Verification items for the finished model (mm, model axes). Face numbers are marked on the shaded views. A direction names the side the tool comes from. Round coordinates to 2 decimals unless told otherwise and drop trailing zeros. Write each loop counter-clockwise with the first axis right and the second up, starting at its lowest first coordinate (ties: lowest second). Pieces come first, ordered by that corner, then holes. Notation, with made-up numbers: (50, 38.5) - (83, 38.5) arc R13 ccw to (83, 51.5) - close; hole circle Ø1 at (74.5, -20). An arc over 180 degrees is marked (long way). Write each question's results on one line, items separated by ' | '.
```python
from build123d import *

# Parameters (mm, degrees)
SKETCH1_W           = 31
SKETCH1_H           = 26
BOSS_EXTRUDE1_DEPTH = 16.5
CUT_EXTRUDE1_START  = -6.5
SKETCH3_R           = 1.715784354
CUT_EXTRUDE1_DEPTH  = 8
SKETCH4_W           = 7.501797644
SKETCH4_H           = 16.91664374
CUT_EXTRUDE2_DEPTH  = 14.5


with BuildPart() as part:
    # Sketch1 → Boss-Extrude1 (new body)
    with BuildSketch(Plane.XY):
        with Locations((15.5, 13)):
            Rectangle(SKETCH1_W, SKETCH1_H)
    extrude(amount=BOSS_EXTRUDE1_DEPTH)

    # Sketch3 → Cut-Extrude1 (cut)
    with BuildSketch(Plane.XY.offset(16.5).offset(CUT_EXTRUDE1_START)):
        Polygon((0, 0), (0, 4.632335589), (6.323496347, 4.632335589), (6.323496347, 21.367664411), (0, 21.367664411), (0, 26), (31, 26), (31, 0), align=None)
        with Locations((3.010252107, 2.158101323)):
            Circle(SKETCH3_R, mode=Mode.SUBTRACT)
        with Locations((19.83045716, 2.158101323)):
            Circle(SKETCH3_R, mode=Mode.SUBTRACT)
        with Locations(Location((3.010252107, 23.841898677, 0), (0, 0, 180))):
            Circle(SKETCH3_R, mode=Mode.SUBTRACT)
        with Locations(Location((19.83045716, 23.841898677, 0), (0, 0, 180))):
            Circle(SKETCH3_R, mode=Mode.SUBTRACT)
    extrude(amount=-CUT_EXTRUDE1_DEPTH, mode=Mode.SUBTRACT)

    # Sketch4 → Cut-Extrude2 (cut)
    with BuildSketch(Plane.XY.offset(16.5)):
        with Locations((3.750898822, 13)):
            Rectangle(SKETCH4_W, SKETCH4_H)
    extrude(amount=-CUT_EXTRUDE2_DEPTH, mode=Mode.SUBTRACT)


solid = part.part
```
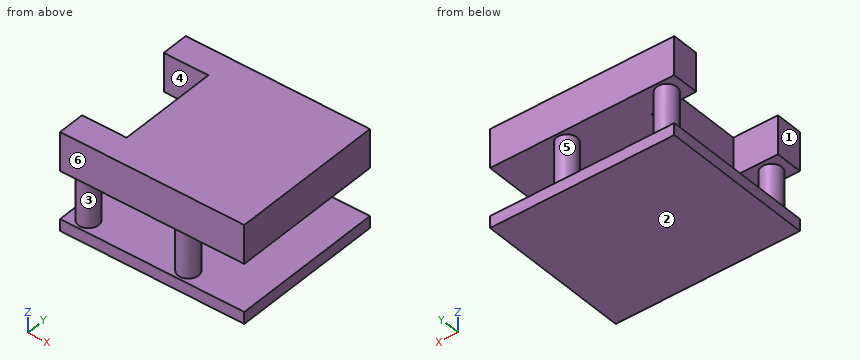
(1) Mould release check, pull along Z, two halves, no side actions. Record for the marked faces 1, 2 and 3: released by +Z, released by -Z, zero draft, split by the parting line, or undercut.
Answer:
face 1: zero draft | face 2: released by -Z | face 3: undercut
(2) Section check D-D (z = 12.25). Record the cut outline in (x, y).
Answer:
outline: (0, 0) - (31, 0) - (31, 26) - (0, 26) - (0, 21.46) - (7.5, 21.46) - (7.5, 4.54) - (0, 4.54) - close
(3) Section check C-C (x = 28). Record the cut outline in (y, z).
Answer:
outline: (0, 0) - (26, 0) - (26, 2) - (0, 2) - close; (0, 10) - (26, 10) - (26, 16.5) - (0, 16.5) - close
(4) Go/stop test with flat-tipped pins: pin 1 Ø1.5 at (x, z) = (25, 3.5) entering from +Y; pin 2 Ø2 at (y, z) = (10.5, 11.5) entering from -X. Record where each tip stops, or that it passes through.
Answer:
pin 1: through | pin 2: x = 7.5
(5) Thickness scan on L1, parallel to Z at x = 24, y = 1.5; L2, parallel to Y at x = 4.5, z = 12; L3, parallel to X at y = 12.5, z = 13. Record the ranges inside material, lowest first.
Answer:
L1: 0 to 2, 10 to 16.5 | L2: 0 to 4.54, 21.46 to 26 | L3: 7.5 to 31
(6) Section check A-A (x = 6). Record the cut outline in (y, z).
Answer:
outline: (0, 0) - (26, 0) - (26, 2) - (0, 2) - close; (0, 10) - (4.54, 10) - (4.54, 16.5) - (0, 16.5) - close; (21.46, 10) - (26, 10) - (26, 16.5) - (21.46, 16.5) - close
(7) Set-up check for the marked faces 4, 5 and 6: record each of +Z, -Z, +X, -X, +Y, -Y from which the full face is reachable in a straight line by a thin tool's end or side.
Answer:
face 4: +Z, -X | face 5: none | face 6: +Z, -Z, +X, -X, -Y
(8) Section check B-B (y = 15.5). Record the cut outline in (x, z).
Answer:
outline: (0, 0) - (31, 0) - (31, 2) - (0, 2) - close; (7.5, 10) - (31, 10) - (31, 16.5) - (7.5, 16.5) - close
